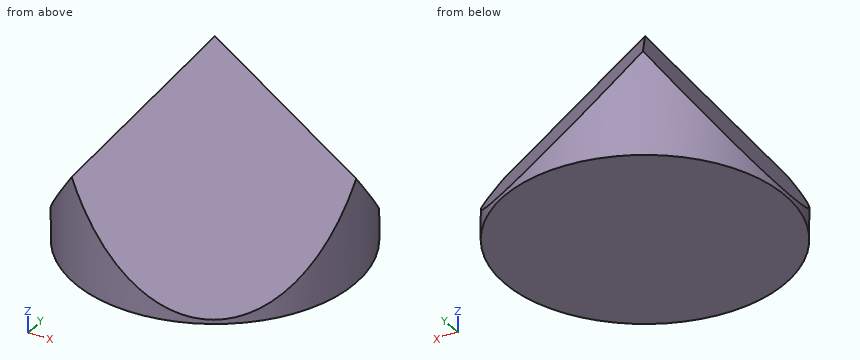
from build123d import *

# Parameters (mm, degrees)
SKETCH_1_R          = 36.25
EXTRUDE_1_DEPTH     = 52.35
CUT_EXTRUDE_1_DEPTH = 39.5
CUT_EXTRUDE_2_DEPTH = 62
CUT_EXTRUDE_3_DEPTH = 53.5


with BuildPart() as part:
    # 草图1 → 凸台-拉伸1 (new body)
    with BuildSketch(Plane.XY):
        Circle(SKETCH_1_R)
    extrude(amount=EXTRUDE_1_DEPTH)

    # 草图2 → 切除-拉伸1 (cut, symmetric)
    with BuildSketch(Plane(origin=(0, 0, 0), x_dir=(1, 0, 0), z_dir=(0, 1, 0))):
        Polygon((0, -52.35), (-40.690324156, 5.182856926), (-40.690324156, -56.656954578), (0, -56.656954578), align=None)
    extrude(amount=CUT_EXTRUDE_1_DEPTH, both=True, mode=Mode.SUBTRACT)

    # 草图4 → 切除-拉伸2 (cut, symmetric)
    with BuildSketch(Plane(origin=(0, 0, 0), x_dir=(0.5, 0.866025404, 0), z_dir=(0.866025404, -0.5, 0))):
        Polygon((0, 52.35), (102.797241837, -92.997060504), (102.797241837, 79.089205692), (0, 79.089205692), align=None)
    extrude(amount=CUT_EXTRUDE_2_DEPTH, both=True, mode=Mode.SUBTRACT)

    # 草图5 → 切除-拉伸3 (cut, symmetric)
    with BuildSketch(Plane(origin=(0, 0, 0), x_dir=(0.5, -0.866025404, 0), z_dir=(-0.866025404, -0.5, 0))):
        Polygon((0, 52.35), (47.788184694, -15.218662816), (47.788184694, 62.081252558), (2.684670532, 62.081252558), align=None)
    extrude(amount=CUT_EXTRUDE_3_DEPTH, both=True, mode=Mode.SUBTRACT)


solid = part.part
Here's how the part is built. I have some questions about the finished solid (model axes, mm). Coordinates: 2 decimals unless noted, no trailing zeros. Loops run counter-clockwise (first coordinate to the right, second up) from the corner with the lowest first, then second, coordinate; pieces in that order, holes last.
1. I need wall thicknesses on L1, parallel to Y at x = -11.5, z = 30; L2, parallel to Z at x = 12, y = 13; L3, parallel to X at y = 18, z = 29. Which ranges of each line are inside material? Lowest first, please.
2. Imagine slicing it at B-B, the plane y = 11.5. Please give me the cut outline in (x, z), and give its area (3 significant figures).
3. Imagine slicing it at C-C, the plane x = 10. Please give me the cut outline in (y, z).
4. Imagine slicing it at D-D, the plane z = 13.5. Please give me the cut outline in (x, y), and give its area (3 significant figures).
5. Imagine slicing it at A-A, the plane z = 22.5. Please give me the cut outline in (x, y), and give its area (3 significant figures).
6. For P1, Ø1, axis at x = -22, y = 5, coming from the +Z side; P2, Ø2, axis at x = -12, y = -25, coming from the +Z side; P3, Ø6, axis at x = -22.5, z = 17, coming from the -Y side, each with a flat end and sliding along its axis, tell me the tip position at first contact or that it passes through.
Taken from the geometry:
1. L1: y = -24.89 to 24.89
1. L2: z = 0 to 27.95
1. L3: x = -16.51 to 1.85
2. outline: (-34.38, 0) - (34.38, 0) - (34.38, 13.96) - (-6.64, 42.96) - (-34.38, 3.74) - close
2. area: 1,820 mm2
3. outline: (-34.84, 0) - (34.84, 0) - (34.84, 2.61) - (0, 45.28) - (-34.84, 2.61) - close
4. outline: (-27.48, -23.65) arc R36.25 ccw to (-6.74, -35.62) - (34.22, -11.97) arc R36.25 ccw to (34.22, 11.97) - (-6.74, 35.62) arc R36.25 ccw to (-27.48, 23.65) - close
4. area: 3,280 mm2
5. outline: (-21.11, -29.47) arc R36.25 ccw to (-14.96, -33.02) - (36.08, -3.55) arc R36.25 ccw to (36.08, 3.55) - (-14.96, 33.02) arc R36.25 ccw to (-21.11, 29.47) - close
5. area: 2,250 mm2
6. P1: stops at z = 21.95
6. P2: stops at z = 31.64
6. P3: stops at y = -30.56
